from build123d import *

# Parameters (mm, degrees)
F0_W     = 37.211
F0_H     = 39.37
F1_DEPTH = 5.207
F2_W     = 35.56
F2_H     = 8.89
F3_DEPTH = 39.37
F4_R     = 0.76199


# Not quite as in the source:
# - a fillet or chamfer is up to 0.001 mm smaller than in the source, because OpenCascade refuses the exact size


with BuildPart() as f1:
    # F0 (on Front) → F1 (new body, symmetric)
    with BuildSketch(Plane.XZ):
        Rectangle(F0_W, F0_H)
    extrude(amount=F1_DEPTH, both=True)

    # F2 (on face) → F3 (cut)
    with BuildSketch(Plane.XY.offset(19.685)):
        Rectangle(F2_W, F2_H)
    extrude(amount=-F3_DEPTH, mode=Mode.SUBTRACT)

    # F4 (radius 0.762 in the source; OpenCascade refuses exactly that, so slightly less here)
    f4_edges = [f1.edges().sort_by_distance(p)[0] for p in [
        (18.6055, 0, -19.685),
        (0, -5.207, -19.685),
        (0, 5.207, -19.685),
        (-18.6055, 0, -19.685),
    ]]
    fillet(f4_edges, radius=F4_R)


solid = f1.part
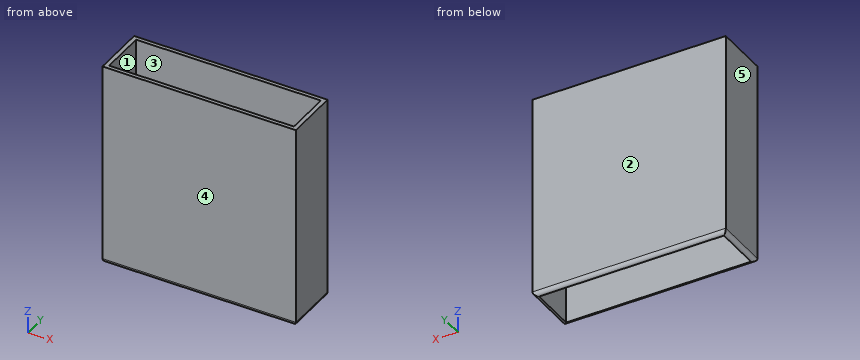
Here's how the part is built. I have some questions about the finished solid (model axes, mm). Face numbers are marked on the shaded views. A direction names the side the tool comes from. Round coordinates to 2 decimals unless told otherwise and drop trailing zeros. Order: outer loops, then holes, each group sorted by start corner. A loop starts at its lowest first (then second) coordinate and runs counter-clockwise, first axis right, second up. Notation, with made-up numbers: M -31,51.5 L 21,51.5 A22 ccw 21,65.5 Z; hole C 78.5,22.25 d3. An arc over 180 degrees is marked long. Return JSON: item names as keys, results as strings. Group by question number.
1. Please list where these lines run through material, in increasing order: probe 1 along X at (y, z) = (0.25, -1); probe 2 along Y at (x, z) = (6, -10) (3 decimals); probe 3 along Z at (x, y) = (-0.5, 4.5) (3 decimals).
2. I'm going to push a flat-ended pin straight in: pin 1 Ø1 at (x, y) = (14.5, -3) entering from -Z. Where does the tip first touch, or does it pass through?
3. If we mould it in two halves opening along Y, with no side actions, what happens to the marked faces 3, 4 and 5? For each: pulls with the +Y half, pulls with the -Y half, needs draft (parallel to the pull), parting line crosses it, or undercut.
4. On a 3-axis mill with a long thin cutter (end or side, diameter ignored), from which of +Z, -Z, +X, -X, +Y, -Y can I reach the whole of each face in a straight line? I mean the marked faces 1 and 2. Say none if no direction works.
5. If we section it at B-B on z = -9: List the corners of the cut face in (x, y) for me (1 decimal).
Reply:
{
 "1": {"probe 1": "-18.61 to -17.78, 17.78 to 18.61", "probe 2": "-5.207 to -4.445, 4.445 to 5.207", "probe 3": "-19.683 to 19.685"},
 "2": {"pin 1": "through"},
 "3": {"face 3": "undercut", "face 4": "pulls with the -Y half", "face 5": "needs draft"},
 "4": {"face 1": "+Z, -Z", "face 2": "+Z, -Z, +X, -X, +Y"},
 "5": {"outline": "M -18.6,-5.2 L 18.6,-5.2 L 18.6,5.2 L -18.6,5.2 Z; hole M -17.8,-4.4 L 17.8,-4.4 L 17.8,4.4 L -17.8,4.4 Z"}
}
